```python
from build123d import *

# Parameters (mm, degrees)
SKETCH_1_R      = 2.5
SKETCH_1_R_2    = 3.5
EXTRUDE_1_DEPTH = 100


with BuildPart() as part:
    # 草图1 → 凸台-拉伸1 (new body)
    with BuildSketch(Plane.XY):
        Polygon((-29.877197952, 10.487377279), (-29.877197952, -1.362622721), (-29.877197952, -13.212622721), (-27.377197952, -13.212622721), (-27.377197952, -10.712622721), (-22.377197952, -10.712622721), (-22.377197952, -13.212622721), (-19.877197952, -13.212622721), (-19.877197952, -19.512622721), (-22.377197952, -19.512622721), (-22.377197952, -22.012622721), (-27.377197952, -22.012622721), (-27.377197952, -19.512622721), (-29.877197952, -19.512622721), (-29.877197952, -31.362622721), (-18.027197952, -31.362622721), (-18.027197952, -28.862622721), (-20.527197952, -28.862622721), (-20.527197952, -23.862622721), (-18.027197952, -23.862622721), (-18.027197952, -21.362622721), (-11.727197952, -21.362622721), (-11.727197952, -23.862622721), (-9.227197952, -23.862622721), (-9.227197952, -28.862622721), (-11.727197952, -28.862622721), (-11.727197952, -31.362622721), (0.122802048, -31.362622721), (11.972802048, -31.362622721), (11.972802048, -28.862622721), (9.472802048, -28.862622721), (9.472802048, -23.862622721), (11.972802048, -23.862622721), (11.972802048, -21.362622721), (18.272802048, -21.362622721), (18.272802048, -23.862622721), (20.772802048, -23.862622721), (20.772802048, -28.862622721), (18.272802048, -28.862622721), (18.272802048, -31.362622721), (30.122802048, -31.362622721), (30.122802048, -19.512622721), (27.622802048, -19.512622721), (27.622802048, -22.012622721), (22.622802048, -22.012622721), (22.622802048, -19.512622721), (20.122802048, -19.512622721), (20.122802048, -13.212622721), (22.622802048, -13.212622721), (22.622802048, -10.712622721), (27.622802048, -10.712622721), (27.622802048, -13.212622721), (30.122802048, -13.212622721), (30.122802048, -1.362622721), (30.122802048, 10.487377279), (27.622802048, 10.487377279), (27.622802048, 7.987377279), (22.622802048, 7.987377279), (22.622802048, 10.487377279), (20.122802048, 10.487377279), (20.122802048, 16.787377279), (22.622802048, 16.787377279), (22.622802048, 19.287377279), (27.622802048, 19.287377279), (27.622802048, 16.787377279), (30.122802048, 16.787377279), (30.122802048, 28.637377279), (18.272802048, 28.637377279), (18.272802048, 26.137377279), (20.772802048, 26.137377279), (20.772802048, 21.137377279), (18.272802048, 21.137377279), (18.272802048, 18.637377279), (11.972802048, 18.637377279), (11.972802048, 21.137377279), (9.472802048, 21.137377279), (9.472802048, 26.137377279), (11.972802048, 26.137377279), (11.972802048, 28.637377279), (0.122802048, 28.637377279), (-11.727197952, 28.637377279), (-11.727197952, 26.137377279), (-9.227197952, 26.137377279), (-9.227197952, 21.137377279), (-11.727197952, 21.137377279), (-11.727197952, 18.637377279), (-18.027197952, 18.637377279), (-18.027197952, 21.137377279), (-20.527197952, 21.137377279), (-20.527197952, 26.137377279), (-18.027197952, 26.137377279), (-18.027197952, 28.637377279), (-29.877197952, 28.637377279), (-29.877197952, 16.787377279), (-27.377197952, 16.787377279), (-27.377197952, 19.287377279), (-22.377197952, 19.287377279), (-22.377197952, 16.787377279), (-19.877197952, 16.787377279), (-19.877197952, 10.487377279), (-22.377197952, 10.487377279), (-22.377197952, 7.987377279), (-27.377197952, 7.987377279), (-27.377197952, 10.487377279), align=None)
        with Locations((-14.877197952, 13.637377279)):
            Circle(SKETCH_1_R, mode=Mode.SUBTRACT)
        with Locations((-25.202197952, 23.962377279)):
            Circle(SKETCH_1_R_2, mode=Mode.SUBTRACT)
        with Locations((15.122802048, 13.637377279)):
            Circle(SKETCH_1_R, mode=Mode.SUBTRACT)
        with Locations((25.447802048, 23.962377279)):
            Circle(SKETCH_1_R_2, mode=Mode.SUBTRACT)
        with Locations((-14.877197952, -16.362622721)):
            Circle(SKETCH_1_R, mode=Mode.SUBTRACT)
        with Locations((-25.202197952, -26.687622721)):
            Circle(SKETCH_1_R_2, mode=Mode.SUBTRACT)
        with Locations((15.122802048, -16.362622721)):
            Circle(SKETCH_1_R, mode=Mode.SUBTRACT)
        with Locations((25.447802048, -26.687622721)):
            Circle(SKETCH_1_R_2, mode=Mode.SUBTRACT)
        with BuildLine():
            Line((0.122802048, 26.337377279), (-5.227197952, 26.337377279))
            ThreePointArc((-5.227197952, 26.337377279), (-6.994964905, 25.605144232), (-7.727197952, 23.837377279))
            Line((-7.727197952, 23.837377279), (-7.727197952, 19.637377279))
            Line((-7.727197952, 19.637377279), (-11.532834307, 15.831740924))
            ThreePointArc((-11.532834307, 15.831740924), (-12.048770828, 10.808950154), (-17.071561598, 10.293013634))
            Line((-17.071561598, 10.293013634), (-20.877197952, 6.487377279))
            Line((-20.877197952, 6.487377279), (-25.077197952, 6.487377279))
            ThreePointArc((-25.077197952, 6.487377279), (-26.844964905, 5.755144232), (-27.577197952, 3.987377279))
            Line((-27.577197952, 3.987377279), (-27.577197952, -6.712622721))
            ThreePointArc((-27.577197952, -6.712622721), (-26.844964905, -8.480389674), (-25.077197952, -9.212622721))
            Line((-25.077197952, -9.212622721), (-20.877197952, -9.212622721))
            Line((-20.877197952, -9.212622721), (-17.071561598, -13.018259076))
            ThreePointArc((-17.071561598, -13.018259076), (-12.048770828, -13.534195596), (-11.532834307, -18.556986366))
            Line((-11.532834307, -18.556986366), (-7.727197952, -22.362622721))
            Line((-7.727197952, -22.362622721), (-7.727197952, -26.562622721))
            ThreePointArc((-7.727197952, -26.562622721), (-6.994964905, -28.330389674), (-5.227197952, -29.062622721))
            Line((-5.227197952, -29.062622721), (0.122802048, -29.062622721))
            Line((0.122802048, -29.062622721), (5.472802048, -29.062622721))
            ThreePointArc((5.472802048, -29.062622721), (7.240569001, -28.330389674), (7.972802048, -26.562622721))
            Line((7.972802048, -26.562622721), (7.972802048, -22.362622721))
            Line((7.972802048, -22.362622721), (11.778438402, -18.556986366))
            ThreePointArc((11.778438402, -18.556986366), (12.294374923, -13.534195596), (17.317165693, -13.018259076))
            Line((17.317165693, -13.018259076), (21.122802048, -9.212622721))
            Line((21.122802048, -9.212622721), (25.322802048, -9.212622721))
            ThreePointArc((25.322802048, -9.212622721), (27.090569001, -8.480389674), (27.822802048, -6.712622721))
            Line((27.822802048, -6.712622721), (27.822802048, 3.987377279))
            ThreePointArc((27.822802048, 3.987377279), (27.090569001, 5.755144232), (25.322802048, 6.487377279))
            Line((25.322802048, 6.487377279), (21.122802048, 6.487377279))
            Line((21.122802048, 6.487377279), (17.317165693, 10.293013634))
            ThreePointArc((17.317165693, 10.293013634), (12.294374923, 10.808950154), (11.778438402, 15.831740924))
            Line((11.778438402, 15.831740924), (7.972802048, 19.637377279))
            Line((7.972802048, 19.637377279), (7.972802048, 23.837377279))
            ThreePointArc((7.972802048, 23.837377279), (7.240569001, 25.605144232), (5.472802048, 26.337377279))
            Line((5.472802048, 26.337377279), (0.122802048, 26.337377279))
        make_face(mode=Mode.SUBTRACT)
    extrude(amount=EXTRUDE_1_DEPTH)


solid = part.part
```
The listing builds one solid part. Answer for the finished solid, in the listing's coordinates (mm). A direction names the side the tool comes from. Coordinates: 2 decimals unless noted, no trailing zeros. Write each loop counter-clockwise with the first axis right and the second up, starting at its lowest first coordinate (ties: lowest second). Pieces come first, ordered by that corner, then holes.
Q1. Section A-A, the plane x = -3 is taken. Write down the section's boundary in (y, z), then the cut area to 3 significant figures.
Returned:
outline: (-31.36, 0) - (-29.06, 0) - (-29.06, 100) - (-31.36, 100) - close; (26.34, 0) - (28.64, 0) - (28.64, 100) - (26.34, 100) - close
area: 460 mm2
Q2. Section D-D, the plane z = 38 is taken. Give the number of separate pieces and of enclosed holes in the cut face, then the cut area to 3 significant figures.
Returned:
separate pieces: 1
enclosed holes: 9
area: 910 mm2
Q3. Given P1, Ø12, axis at y = -16.5, z = 76.5, coming from the -X side, flat-ended and moving along its own axis, determine where the tip first touches the part or whether it passes through.
Returned:
P1: stops at x = -29.88
Q4. Section C-C, the plane x = 24 is taken. Write down the section's boundary in (y, z).
Returned:
outline: (-31.36, 0) - (-29.87, 0) - (-29.87, 100) - (-31.36, 100) - close; (-23.5, 0) - (-22.01, 0) - (-22.01, 100) - (-23.5, 100) - close; (-10.71, 0) - (-9.21, 0) - (-9.21, 100) - (-10.71, 100) - close; (6.49, 0) - (7.99, 0) - (7.99, 100) - (6.49, 100) - close; (19.29, 0) - (20.78, 0) - (20.78, 100) - (19.29, 100) - close; (27.15, 0) - (28.64, 0) - (28.64, 100) - (27.15, 100) - close
Q5. Which of the six approach directions +Z, -Z, +X, -X, +Y, -Y give full straight-line access (tool end or side, diameter ignored) to faces 1 (the flat face through (18.273, -30, 49)), 2 (the flat face through (29, -19.513, 49)), 3 (the flat face through (22.623, -12, 49)), 4 (the flat face through (24, 28.637, 49))?
Returned:
face 1: +Z, -Z, -Y
face 2: +Z, -Z, +X
face 3: +Z, -Z
face 4: +Z, -Z, +X, -X, +Y
Q6. Find the intervals of material crossed by line 1 along Y through (x, z) = (-21.5, 68.5); line 2 along Y through (x, z) = (-4.5, 64.5); line 3 along X through (y, z) = (-1, 23), in increasing order.
Returned:
line 1: y = -31.36 to -19.51, -13.21 to -9.21, 6.49 to 10.49, 16.79 to 28.64
line 2: y = -31.36 to -29.06, 26.34 to 28.64
line 3: x = -29.88 to -27.58, 27.82 to 30.12
Q7. Section B-B, the plane y = -15 is taken. Write down the section's boundary in (x, z), then the cut area to 3 significant figures.
Returned:
outline: (-19.88, 0) - (-16.97, 0) - (-16.97, 100) - (-19.88, 100) - close; (-12.78, 0) - (-11.12, 0) - (-11.12, 100) - (-12.78, 100) - close; (11.36, 0) - (13.03, 0) - (13.03, 100) - (11.36, 100) - close; (17.22, 0) - (20.12, 0) - (20.12, 100) - (17.22, 100) - close
area: 914 mm2
Q8. The mould has two halves that part along X. Classify faces 5 (the flat face through (0, 26.337, 49)), 6 (the flat face through (-29, 10.487, 49)), 7 (the flat face through (30.123, 23, 49)): released by +X, released by -X, zero draft, split by the parting line, or undercut.
Returned:
face 5: undercut
face 6: zero draft
face 7: released by +X
